The listing builds one solid part. Answer for the finished solid, in the listing's coordinates (mm). A direction names the side the tool comes from. Give positions to 0.01 mm unless a question says otherwise; leave off trailing zeros. Write each loop counter-clockwise with the first axis right and the second up, starting at its lowest first coordinate (ties: lowest second). Pieces come first, ordered by that corner, then holes. Notation, with made-up numbers: (63.5, 10.25) - (97.5, 10.25) arc R20 ccw to (97.5, 21.25) - close; hole circle Ø1 at (-29, 8.5). An arc over 180 degrees is marked (long way). Answer as CSV lines item,"result". Start each with the question number.
(1) For a pull along Z with two mould halves and no side action, classify faces 3 (the face through (20.7, 10.37, -20.63)), 4 (the face through (0, 3, 0)), 5 (the face through (0, 9, 15.3)), 6 (the face through (20.63, 10.37, 20.7)) as pulls with the +Z half, pulls with the -Z half, needs draft (parallel to the pull), parting line crosses it, or undercut.
(2) Find section A-A (x = -38). Write down the section's boundary in (y, z).
(3) Find section B-B (z = -34.5). Write down the section's boundary in (x, y), then the cut area to 3 significant figures.
(4) Straight lines are drawn through the part: probe 1 along Y at (x, z) = (-33.5, 13); probe 2 along Z at (x, y) = (-1.5, 7.5); probe 3 along Z at (x, y) = (-15, 6). For each, find the intervals that lie inside material, in ascending order.
(5) Each of these flat-tipped pins is pushed along its axis until it touches: pin 1 Ø3 at (x, z) = (9.5, 18.5) entering from -Y; pin 2 Ø1 at (y, z) = (1.5, 12) entering from +X; pin 3 Ø5 at (x, y) = (26, 5.5) entering from +Z; pin 4 Ø4 at (y, z) = (12.5, -13.5) entering from +X. Where does it stop, or does it pass through?
(6) For faces 1 (the face through (21.415, 5.443, -21.337)), 2 (the face through (0, 5, -24)), determine the directions among +Z, -Z, +X, -X, +Y, -Y from which every point of the face is accessible in a straight line to the end or side of a thin tool.
from build123d import *
from OCP.BRepFilletAPI import BRepFilletAPI_MakeChamfer

# Parameters (mm, degrees)
BOSS_EXTRUDE1_DEPTH = 5
BOSS_EXTRUDE2_START = 5
BOSS_EXTRUDE2_DEPTH = 10
BOSS_EXTRUDE2_TAPER = 10
CUT_EXTRUDE1_START  = 3
SKETCH1_5_W         = 30.6
SKETCH1_5_H         = 30.6
CUT_EXTRUDE1_DEPTH  = 12
CHAMFER1_SIZE       = 0.5
CHAMFER1_SIZE2      = 0.616401526


with BuildPart() as part:
    # Sketch1 → Boss-Extrude1 (new body)
    with BuildSketch(Plane(origin=(0, 0, 0), x_dir=(1, 0, 0), z_dir=(0, 1, 0))):
        with BuildLine():
            Line((7.071067812, -42.928932188), (42.928932188, -7.071067812))
            ThreePointArc((42.928932188, -7.071067812), (45.857864376, 0), (42.928932188, 7.071067812))
            Line((42.928932188, 7.071067812), (7.071067812, 42.928932188))
            ThreePointArc((7.071067812, 42.928932188), (0, 45.857864376), (-7.071067812, 42.928932188))
            Line((-7.071067812, 42.928932188), (-42.928932188, 7.071067812))
            ThreePointArc((-42.928932188, 7.071067812), (-45.857864376, 0), (-42.928932188, -7.071067812))
            Line((-42.928932188, -7.071067812), (-7.071067812, -42.928932188))
            ThreePointArc((-7.071067812, -42.928932188), (0, -45.857864376), (7.071067812, -42.928932188))
        make_face()
    extrude(amount=BOSS_EXTRUDE1_DEPTH)

    # Sketch1<4> → Boss-Extrude2 (add)
    with BuildSketch(Plane(origin=(0, 0, 0), x_dir=(1, 0, 0), z_dir=(0, 1, 0)).offset(BOSS_EXTRUDE2_START)):
        with BuildLine():
            ThreePointArc((17.8, -22.8), (21.335533906, -21.335533906), (22.8, -17.8))
            Line((22.8, -17.8), (22.8, 17.8))
            ThreePointArc((22.8, 17.8), (21.335533906, 21.335533906), (17.8, 22.8))
            Line((17.8, 22.8), (-17.8, 22.8))
            ThreePointArc((-17.8, 22.8), (-21.335533906, 21.335533906), (-22.8, 17.8))
            Line((-22.8, 17.8), (-22.8, -17.8))
            ThreePointArc((-22.8, -17.8), (-21.335533906, -21.335533906), (-17.8, -22.8))
            Line((-17.8, -22.8), (17.8, -22.8))
        make_face()
    extrude(amount=BOSS_EXTRUDE2_DEPTH, taper=BOSS_EXTRUDE2_TAPER)

    # Sketch1<5> → Cut-Extrude1 (cut)
    with BuildSketch(Plane(origin=(0, 0, 0), x_dir=(1, 0, 0), z_dir=(0, 1, 0)).offset(CUT_EXTRUDE1_START)):
        Rectangle(SKETCH1_5_W, SKETCH1_5_H)
    extrude(amount=CUT_EXTRUDE1_DEPTH, mode=Mode.SUBTRACT)

    # Chamfer1: one chamfer whose edges measure the first distance from different faces: ONE call of the kernel's chamfer builder (chamfer() names one face for all edges)
    chamfer1_edges_1 = [part.edges().sort_by_distance(p)[0] for p in [
        (0, 5, -45.857864376),
        (-25, 5, -25),
        (-45.857864376, 5, 0),
        (-25, 5, 25),
        (0, 5, 45.857864376),
        (25, 5, 25),
        (45.857864376, 5, 0),
        (25, 5, -25),
    ]]
    chamfer1_edges_2 = [part.edges().sort_by_distance(p)[0] for p in [
        (21.335533906, 5, -21.335533906),
        (-21.335533906, 5, -21.335533906),
        (-22.8, 5, 0),
        (-21.335533906, 5, 21.335533906),
        (0, 5, 22.8),
        (21.335533906, 5, 21.335533906),
        (22.8, 5, 0),
        (0, 5, -22.8),
    ]]
    chamfer1_side_2 = [part.faces().sort_by_distance(p)[0] for p in [
        (24.082842712, 5, 24.082842712),
    ]]
    chamfer1 = BRepFilletAPI_MakeChamfer(part.part.solid().wrapped)
    for e in chamfer1_edges_1:
        chamfer1.Add(CHAMFER1_SIZE, e.wrapped)
    for e in chamfer1_edges_2:
        chamfer1.Add(CHAMFER1_SIZE, CHAMFER1_SIZE2, e.wrapped, chamfer1_side_2[0].wrapped)  # the first distance lies on this face
    add(Compound.cast(chamfer1.Shape()), mode=Mode.REPLACE)


solid = part.part
Result set:
1,face 3,"pulls with the -Z half"
1,face 4,"undercut"
1,face 5,"undercut"
1,face 6,"pulls with the +Z half"
2,outline,"(0, -12) - (4.5, -12) - (5, -11.29) - (5, 11.29) - (4.5, 12) - (0, 12) - close"
3,outline,"(-15.5, 0) - (15.5, 0) - (15.5, 4.5) - (14.79, 5) - (-14.79, 5) - (-15.5, 4.5) - close"
3,area,"155 mm^2"
4,probe 1,"0 to 5"
4,probe 2,"-22.36 to -15.3, 15.3 to 22.36"
4,probe 3,"-22.62 to -15.3, 15.3 to 22.62"
5,pin 1,"y = 0"
5,pin 2,"x = 38.5"
5,pin 3,"z = 26.29"
5,pin 4,"x = 21.83"
6,face 1,"-Z, +X, +Y"
6,face 2,"+Y"
